For this review, take the finished solid that the model builds, in its own axes (mm). Give positions to 0.01 mm unless a question says otherwise; leave off trailing zeros. Write each loop counter-clockwise with the first axis right and the second up, starting at its lowest first coordinate (ties: lowest second). Pieces come first, ordered by that corner, then holes.
1) We need section A-A on x = 19.5. Give the boundary of the cut face in (y, z), and give its area (3 significant figures).
2) Wall thickness on line 1 along Z through (x, y) = (77, 86); line 2 along Y through (x, z) = (164.5, -0.4): over which ranges is each line inside the solid? List them lowest first.
3) We need section B-B on y = 28.5. Give the boundary of the cut face in (x, z).
4) We need section D-D on x = 154.5. Give the boundary of the cut face in (y, z).
5) We need section C-C on z = -0.95. Give the boundary of the cut face in (x, y).
6) For P1, Ø1, axis at x = 91, z = -1, coming from the -Y side; P2, Ø1.5, axis at x = 58, y = 90, coming from the +Z side; P3, Ø1.6, axis at y = 161.5, z = -1, coming from the -X side, all flat-tipped, find the tip position at first contact; note any pin that passes through.
from build123d import *

# Parameters (mm, degrees)
SKETCH_1_W        = 209
SKETCH_1_H        = 168
SKETCH_1_W_2      = 201.5
SKETCH_1_H_2      = 152.5
EXTRUDE_1_1_DEPTH = 3
SKETCH_1_3_W      = 201.5
SKETCH_1_3_H      = 152.5
EXTRUDE_1_2_DEPTH = 2.9
SKETCH_3_W        = 150.5
SKETCH_3_H        = 9
EXTRUDE_2_1_DEPTH = 2


with BuildPart() as part:
    # 草图1 → 1-1 (new body)
    with BuildSketch(Plane.XY):
        with Locations((104.5, 84)):
            Rectangle(SKETCH_1_W, SKETCH_1_H)
        with Locations((105.75, 82.75)):
            Rectangle(SKETCH_1_W_2, SKETCH_1_H_2, mode=Mode.SUBTRACT)
    extrude(amount=EXTRUDE_1_1_DEPTH)

    # 草图1<3> → 1-2 (add)
    with BuildSketch(Plane.XY):
        with Locations((105.75, 82.75)):
            Rectangle(SKETCH_1_3_W, SKETCH_1_3_H)
    extrude(amount=EXTRUDE_1_2_DEPTH)

    # 草图3 → 2-1 (add)
    with BuildSketch(Plane(origin=(0, 0, 0), x_dir=(-1, 0, 0), z_dir=(0, 0, -1))):
        with Locations((-108.25, 163.5)):
            Rectangle(SKETCH_3_W, SKETCH_3_H)
    extrude(amount=EXTRUDE_2_1_DEPTH)


solid = part.part
Results list:
1. outline: (0, 0) - (168, 0) - (168, 3) - (159, 3) - (159, 2.9) - (6.5, 2.9) - (6.5, 3) - (0, 3) - close
1. area: 489 mm2
2. line 1: z = 0 to 2.9
2. line 2: y = 159 to 168
3. outline: (0, 0) - (209, 0) - (209, 3) - (206.5, 3) - (206.5, 2.9) - (5, 2.9) - (5, 3) - (0, 3) - close
4. outline: (0, 0) - (159, 0) - (159, -2) - (168, -2) - (168, 3) - (159, 3) - (159, 2.9) - (6.5, 2.9) - (6.5, 3) - (0, 3) - close
5. outline: (33, 159) - (183.5, 159) - (183.5, 168) - (33, 168) - close
6. P1: stops at y = 159
6. P2: stops at z = 2.9
6. P3: stops at x = 33
